The figure shows three views and two pictorial views of one solid part (mm, origin at its lowest corner). Answer the questions. A direction names the side the tool comes from. Give positions to 0.01 mm unless a question says otherwise; leave off trailing zeros. Write each loop counter-clockwise with the first axis right and the second up, starting at its lowest first coordinate (ties: lowest second). Pieces come first, ordered by that corner, then holes. Notation, with made-up numbers: (5.5, 88) -> (26.5, 88) arc R30 ccw to (26.5, 125) -> close; hole circle Ø6 at (81.25, -28). An arc over 180 degrees is marked (long way). Answer as CSV lines item,"result". Start each with the question number.
1. A tool of negligible diameter and unlimited length cuts with its end or side. For the marked faces 1 and 2, from which of +Z, -Z, +X, -X, +Y, -Y can it reach the whole face along a straight path? Write none if from no direction.
2. The part is cut by section D-D, the plane z = 12. Determine the outline of the cut face in (x, y).
3. The part is cut by section A-A, the plane y = 33. Determine the outline of the cut face in (x, z), and give its area (3 significant figures).
4. For a pull along Y with two mould halves and no side action, classify the marked faces 3, 4 and 5 as pulls with the +Y half, pulls with the -Y half, needs draft (parallel to the pull), parting line crosses it, or undercut.
5. The part is cut by section B-B, the plane z = 51.5. Determine the outline of the cut face in (x, y).
6. Find the intervals of material crossed by line 1 (Z direction, x = 8.75, y = 15.5); line 2 (X direction, y = 41.5, z = 42.5); line 3 (Z direction, x = 20.75, y = 29.5), in increasing order.
7. Given pin 1 (5.5 mm diameter, centred on x = 5, y = 15.5, fed in from +Z); pin 2 (4 mm diameter, centred on y = 11, z = 58, fed in from -X), each flat-ended and moving along its own axis, determine where each tip first touches the part or whether it passes through.
8. The part is cut by section C-C, the plane x = 8.5. Determine the outline of the cut face in (y, z).
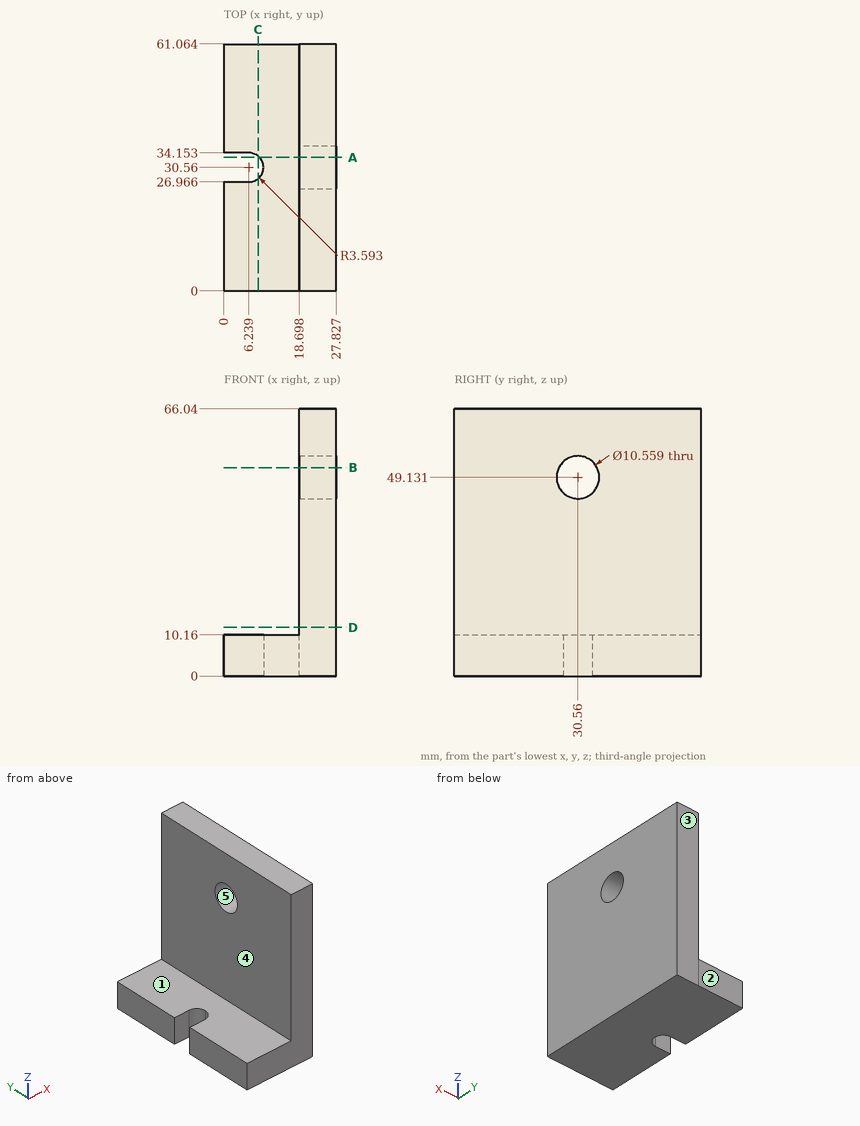
Results found:
1,face 1,"+Z, -X, +Y, -Y"
1,face 2,"+Z, -Z, +X, -X, +Y"
2,outline,"(18.7, 0) -> (27.83, 0) -> (27.83, 61.06) -> (18.7, 61.06) -> close"
3,outline,"(8.88, 0) -> (27.83, 0) -> (27.83, 44.45) -> (18.7, 44.45) -> (18.7, 10.16) -> (8.88, 10.16) -> close; (18.7, 53.81) -> (27.83, 53.81) -> (27.83, 66.04) -> (18.7, 66.04) -> close"
3,area,"617 mm²"
4,face 3,"pulls with the +Y half"
4,face 4,"needs draft"
4,face 5,"undercut"
5,outline,"(18.7, 0) -> (27.83, 0) -> (27.83, 25.84) -> (18.7, 25.84) -> close; (18.7, 35.28) -> (27.83, 35.28) -> (27.83, 61.06) -> (18.7, 61.06) -> close"
6,line 1,"z = 0 to 10.16"
6,line 2,"x = 18.7 to 27.83"
6,line 3,"z = 0 to 43.96, 54.3 to 66.04"
7,pin 1,"stops at z = 10.16"
7,pin 2,"stops at x = 18.7"
8,outline,"(0, 0) -> (27.77, 0) -> (27.77, 10.16) -> (0, 10.16) -> close; (33.35, 0) -> (61.06, 0) -> (61.06, 10.16) -> (33.35, 10.16) -> close"
